Part model, mm, in its own coordinate system. Give positions to 0.01 mm unless a question says otherwise; leave off trailing zeros. Order: outer loops, then holes, each group sorted by start corner. A loop starts at its lowest first (then second) coordinate and runs counter-clockwise, first axis right, second up. Notation, with made-up numbers: M -13.5,20 L -4.5,20 A35 ccw -4.5,59 Z; hole C 88.25,11.5 d4. An arc over 180 degrees is marked long. Write each question's results on one line, items separated by ' | '. Start each with the question number.
from build123d import *

# Parameters (mm, degrees)
SKETCH1_W           = 313
SKETCH1_H           = 342
BOSS_EXTRUDE1_DEPTH = 6.35
SKETCH3_W           = 22
SKETCH3_H           = 155.14040353
SKETCH3_R           = 2.5
BOSS_EXTRUDE2_DEPTH = 6.35
SKETCH2_R           = 2.5
CUT_EXTRUDE1_DEPTH  = 7.35
SKETCH4_R           = 3.5
CUT_EXTRUDE2_DEPTH  = 7.35
SKETCH5_R           = 2
SKETCH5_R_2         = 1.5
SKETCH5_R_3         = 1.05
SKETCH5_R_4         = 2.5
CUT_EXTRUDE3_DEPTH  = 7.35


with BuildPart() as part:
    # Sketch1 → Boss-Extrude1 (new body)
    with BuildSketch(Plane(origin=(0, 0, 0), x_dir=(1, 0, 0), z_dir=(0, 1, 0))):
        Rectangle(SKETCH1_W, SKETCH1_H)
    extrude(amount=-BOSS_EXTRUDE1_DEPTH)

    # Sketch3 → Boss-Extrude2 (add)
    with BuildSketch(Plane(origin=(0, 0, 0), x_dir=(1, 0, 0), z_dir=(0, 1, 0))):
        with Locations((167.5, 9)):
            Rectangle(SKETCH3_W, SKETCH3_H)
        with Locations((166.5, 9)):
            Circle(SKETCH3_R, mode=Mode.SUBTRACT)
        with Locations((166.5, -41.8)):
            Circle(SKETCH3_R, mode=Mode.SUBTRACT)
        with Locations((166.5, 59.8)):
            Circle(SKETCH3_R, mode=Mode.SUBTRACT)
    extrude(amount=-BOSS_EXTRUDE2_DEPTH)

    # Sketch2 → Cut-Extrude1 (cut, through all)
    with BuildSketch(Plane(origin=(0, 0, 0), x_dir=(1, 0, 0), z_dir=(0, 1, 0))):
        with Locations((0, -123)):
            Circle(SKETCH2_R)
        with Locations((-70, -123)):
            Circle(SKETCH2_R)
        with Locations((70, -123)):
            Circle(SKETCH2_R)
        with Locations((-70, 141)):
            Circle(SKETCH2_R)
        with Locations((0, 141)):
            Circle(SKETCH2_R)
        with Locations((70, 141)):
            Circle(SKETCH2_R)
    extrude(amount=-CUT_EXTRUDE1_DEPTH, mode=Mode.SUBTRACT)

    # Sketch4 → Cut-Extrude2 (cut, through all)
    with BuildSketch(Plane(origin=(0, 0, 0), x_dir=(1, 0, 0), z_dir=(0, 1, 0))):
        with Locations((133.64, -142.84)):
            Circle(SKETCH4_R)
        with Locations((108.24, -142.84)):
            Circle(SKETCH4_R)
    cut_extrude2 = extrude(amount=-CUT_EXTRUDE2_DEPTH, mode=Mode.SUBTRACT)

    # Mirror1: Cut-Extrude2 across plane
    add(cut_extrude2.mirror(Plane(origin=(0, 0, -9), x_dir=(1, 0, 0), z_dir=(0, 0, -1))), mode=Mode.SUBTRACT)

    # Sketch5 → Cut-Extrude3 (cut, through all)
    with BuildSketch(Plane(origin=(0, 0, 0), x_dir=(1, 0, 0), z_dir=(0, 1, 0))):
        with Locations((97.385625988, 118.365529647)):
            Circle(SKETCH5_R)
        with Locations((22.33428931, 118.365529647)):
            Circle(SKETCH5_R)
        with Locations((120.259039894, -98.018672219)):
            Circle(SKETCH5_R_2)
        with Locations((34.259039894, -98.018672219)):
            Circle(SKETCH5_R_2)
        with Locations((34.259039894, 37.981327781)):
            Circle(SKETCH5_R_2)
        with Locations((120.259039894, 37.981327781)):
            Circle(SKETCH5_R_2)
        with Locations((14.259039894, -57.018672219)):
            Circle(SKETCH5_R_3)
        with Locations((-130.740960106, -57.018672219)):
            Circle(SKETCH5_R_3)
        with Locations((14.259039894, 37.981327781)):
            Circle(SKETCH5_R_3)
        with Locations((-130.740960106, 37.981327781)):
            Circle(SKETCH5_R_3)
        with Locations((-85.31571069, 117.980264567)):
            Circle(SKETCH5_R_4)
        with Locations((-124.66571069, 117.980264567)):
            Circle(SKETCH5_R_4)
    extrude(amount=-CUT_EXTRUDE3_DEPTH, mode=Mode.SUBTRACT)


solid = part.part
(1) Probe L1, parallel to X at y = -4, z = 123; L2, parallel to Z at x = -70, y = -4; L3, parallel to Z at x = 133.64, y = -2.25. List the from-to ranges inside material, lowest first.
(2) Saw through at B-B on z = -149. Give the cut face in (x, y).
(3) Saw through at A-A on y = -1.5. Give the number of separate pieces and of enclosed holes in the cut face, plus the area to 3 significant figures.
Taken from the geometry:
1) L1: x = -156.5 to -72.5, -67.5 to -2.5, 2.5 to 67.5, 72.5 to 156.5 | L2: z = -171 to -143.5, -138.5 to 120.5, 125.5 to 171 | L3: z = -171 to -164.34, -157.34 to 139.34, 146.34 to 171
2) outline: M -156.5,-6.35 L 156.5,-6.35 L 156.5,0 L -156.5,0 Z
3) separate pieces: 1 | enclosed holes: 25 | area: 110,000 mm²
